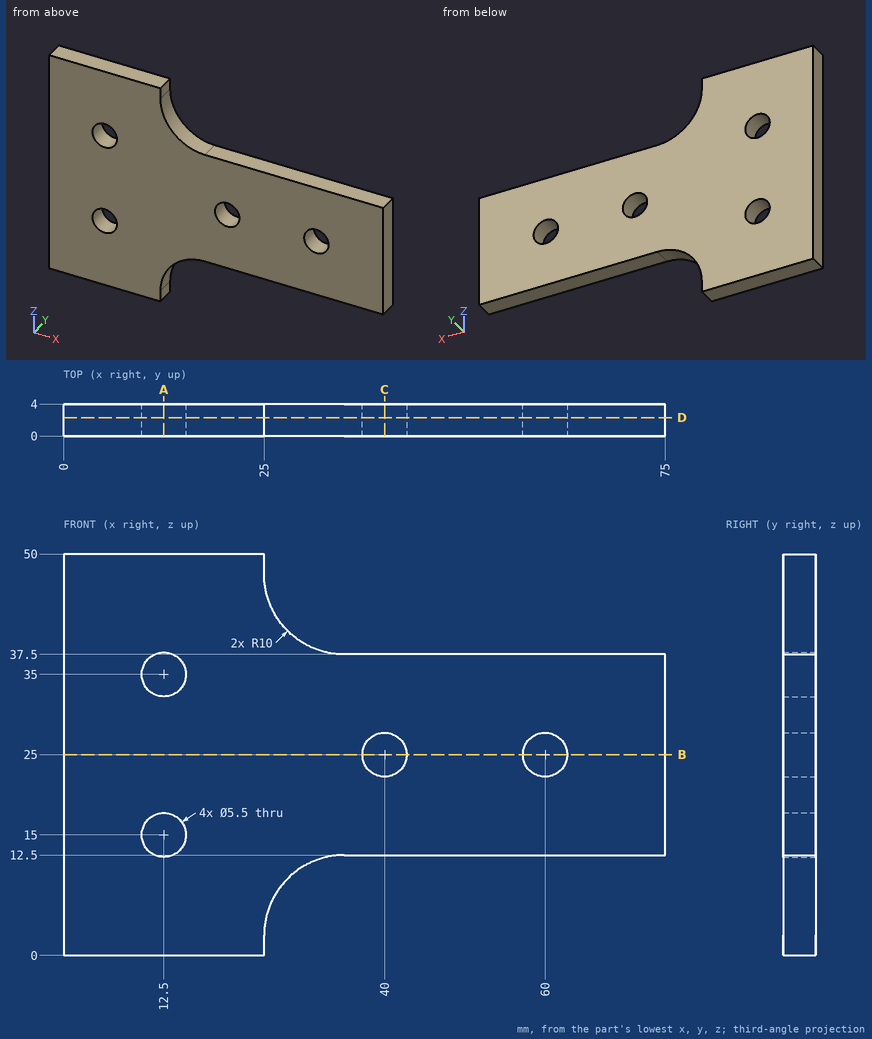
Study the drawing (mm; zero at the part's minimum x, y, z) and answer. Round coordinates to 2 decimals unless told otherwise and drop trailing zeros. Write each loop counter-clockwise with the first axis right and the second up, starting at its lowest first coordinate (ties: lowest second). Pieces come first, ordered by that corner, then holes. Notation, with made-up numbers: (70.25, 41) -> (103.25, 41) arc R8 ccw to (103.25, 54) -> close; hole circle Ø2 at (-39.5, 47.5). An arc over 180 degrees is marked (long way). Write each question's results on one line, items separated by ' | '.
Item 1: Find the intervals of material crossed by line 1 along Z through (x, y) = (12.5, 2.7); line 2 along X through (y, z) = (1, 25); line 3 along Z through (x, y) = (60, 0.95), in increasing order. Write a range as [from, to].
Result set:
line 1: [0, 12.25], [17.75, 32.25], [37.75, 50] | line 2: [0, 37.25], [42.75, 57.25], [62.75, 75] | line 3: [12.5, 22.25], [27.75, 37.5]
Item 2: A cutting plane is placed at B-B, the plane z = 25. Determine the outline of the cut face in (x, y), plus the area to 3 significant figures.
Result set:
outline: (0, 0) -> (37.25, 0) -> (37.25, 4) -> (0, 4) -> close; (42.75, 0) -> (57.25, 0) -> (57.25, 4) -> (42.75, 4) -> close; (62.75, 0) -> (75, 0) -> (75, 4) -> (62.75, 4) -> close | area: 256 mm^2
Item 3: A cutting plane is placed at C-C, the plane x = 40. Determine the outline of the cut face in (y, z).
Result set:
outline: (0, 12.5) -> (4, 12.5) -> (4, 22.25) -> (0, 22.25) -> close; (0, 27.75) -> (4, 27.75) -> (4, 37.5) -> (0, 37.5) -> close
Item 4: A cutting plane is placed at A-A, the plane x = 12.5. Determine the outline of the cut face in (y, z).
Result set:
outline: (0, 0) -> (4, 0) -> (4, 12.25) -> (0, 12.25) -> close; (0, 17.75) -> (4, 17.75) -> (4, 32.25) -> (0, 32.25) -> close; (0, 37.75) -> (4, 37.75) -> (4, 50) -> (0, 50) -> close
Item 5: Flat-ended cylindrical pins translate along their axes: P1, Ø1, axis at x = 45, y = 1, coming from the -Z side; P2, Ø1.2, axis at y = 3, z = 0.5, coming from the +X side; P3, Ø5, axis at x = 12.5, z = 35, coming from the -Y side. Find the tip coordinate at first contact, or state that the pin passes through.
Result set:
P1: z = 12.5 | P2: x = 25 | P3: through
Item 6: A cutting plane is placed at D-D, the plane y = 2.3. Determine the outline of the cut face in (x, z).
Result set:
outline: (0, 0) -> (25, 0) -> (25, 2.5) arc R10 cw to (35, 12.5) -> (75, 12.5) -> (75, 37.5) -> (35, 37.5) arc R10 cw to (25, 47.5) -> (25, 50) -> (0, 50) -> close; hole circle Ø5.5 at (12.5, 15); hole circle Ø5.5 at (12.5, 35); hole circle Ø5.5 at (40, 25); hole circle Ø5.5 at (60, 25)
